from build123d import *

# Parameters (mm, degrees)
SKETCH1_W           = 75
SKETCH1_H           = 75
SKETCH1_R           = 2.625
BOSS_EXTRUDE1_DEPTH = 6.35
FILLET1_R           = 10
SKETCH3_R           = 11.5
SKETCH3_R_2         = 1.75
CUT_EXTRUDE2_DEPTH  = 7.35
SKETCH4_R           = 1.6
CUT_EXTRUDE3_DEPTH  = 7.35


with BuildPart() as part:
    # Sketch1 → Boss-Extrude1 (new body)
    with BuildSketch(Plane(origin=(0, 0, 0), x_dir=(1, 0, 0), z_dir=(0, 1, 0))):
        with Locations((37.5, -37.5)):
            Rectangle(SKETCH1_W, SKETCH1_H)
        with Locations((10, -10)):
            Circle(SKETCH1_R, mode=Mode.SUBTRACT)
        with Locations((45, -10)):
            Circle(SKETCH1_R, mode=Mode.SUBTRACT)
        with Locations((65, -10)):
            Circle(SKETCH1_R, mode=Mode.SUBTRACT)
        with Locations((30, -10)):
            Circle(SKETCH1_R, mode=Mode.SUBTRACT)
    extrude(amount=BOSS_EXTRUDE1_DEPTH)

    # Fillet1
    fillet1_edges = [part.edges().sort_by_distance(p)[0] for p in [
        (75, 3.175, 75),
    ]]
    fillet(fillet1_edges, radius=FILLET1_R)

    # Sketch3 → Cut-Extrude2 (cut, through all)
    with BuildSketch(Plane(origin=(0, 6.35, 0), x_dir=(1, 0, 0), z_dir=(0, 1, 0))):
        with Locations((50, -48)):
            Circle(SKETCH3_R)
        with Locations((34.5, -32.5)):
            Circle(SKETCH3_R_2)
        with Locations((65.5, -32.5)):
            Circle(SKETCH3_R_2)
        with Locations((65.5, -63.5)):
            Circle(SKETCH3_R_2)
        with Locations((34.5, -63.5)):
            Circle(SKETCH3_R_2)
    extrude(amount=-CUT_EXTRUDE2_DEPTH, mode=Mode.SUBTRACT)

    # Sketch4 → Cut-Extrude3 (cut, through all)
    with BuildSketch(Plane(origin=(0, 6.35, 0), x_dir=(1, 0, 0), z_dir=(0, 1, 0))):
        with Locations((22, -15)):
            Circle(SKETCH4_R)
        with Locations((22, -30)):
            Circle(SKETCH4_R)
        with Locations((22, -45)):
            Circle(SKETCH4_R)
        with Locations((22, -60)):
            Circle(SKETCH4_R)
    extrude(amount=-CUT_EXTRUDE3_DEPTH, mode=Mode.SUBTRACT)


solid = part.part
Here's how the part is built. I have some questions about the finished solid (model axes, mm). Round coordinates to 2 decimals unless told otherwise and drop trailing zeros. Order: outer loops, then holes, each group sorted by start corner. A loop starts at its lowest first (then second) coordinate and runs counter-clockwise, first axis right, second up. Notation, with made-up numbers: (16, 83) -> (57, 83) arc R16 cw to (57, 102) -> close; hole circle Ø8 at (-39.75, -8). An arc over 180 degrees is marked (long way). Return JSON: item names as keys, results as strings.
Q1. If we section it at C-C on z = 48: List the corners of the cut face in (x, y) for me, plus the area to 3 significant figures.
Filled sheet:
{"outline": "(0, 0) -> (38.5, 0) -> (38.5, 6.35) -> (0, 6.35) -> close; (61.5, 0) -> (75, 0) -> (75, 6.35) -> (61.5, 6.35) -> close", "area": "330 mm^2"}
Q2. For pin 1 Ø4.5 at (x, z) = (45, 10) entering from -Y (1 decimal), with a flat end and sliding along its axis, tell me the tip position at first contact or that it passes through.
Filled sheet:
{"pin 1": "passes through"}
Q3. If we section it at B-B on z = 10: List the corners of the cut face in (x, y) for me (3 decimals).
Filled sheet:
{"outline": "(0, 0) -> (7.375, 0) -> (7.375, 6.35) -> (0, 6.35) -> close; (12.625, 0) -> (27.375, 0) -> (27.375, 6.35) -> (12.625, 6.35) -> close; (32.625, 0) -> (42.375, 0) -> (42.375, 6.35) -> (32.625, 6.35) -> close; (47.625, 0) -> (62.375, 0) -> (62.375, 6.35) -> (47.625, 6.35) -> close; (67.625, 0) -> (75, 0) -> (75, 6.35) -> (67.625, 6.35) -> close"}
Q4. If we section it at D-D on x = 22: List the corners of the cut face in (y, z) for me, plus the area to 3 significant figures.
Filled sheet:
{"outline": "(0, 0) -> (6.35, 0) -> (6.35, 13.4) -> (0, 13.4) -> close; (0, 16.6) -> (6.35, 16.6) -> (6.35, 28.4) -> (0, 28.4) -> close; (0, 31.6) -> (6.35, 31.6) -> (6.35, 43.4) -> (0, 43.4) -> close; (0, 46.6) -> (6.35, 46.6) -> (6.35, 58.4) -> (0, 58.4) -> close; (0, 61.6) -> (6.35, 61.6) -> (6.35, 75) -> (0, 75) -> close", "area": "395 mm^2"}
Q5. I need wall thicknesses on line 1 along X through (y, z) = (4, 63.5); line 2 along Z through (x, y) = (22, 5.25); line 3 along X through (y, z) = (5.25, 10) (3 decimals). Which ranges of each line are inside material? Lowest first, please. Write a range as from..to.
Filled sheet:
{"line 1": "x = 0..32.75, 36.25..63.75, 67.25..75", "line 2": "z = 0..13.4, 16.6..28.4, 31.6..43.4, 46.6..58.4, 61.6..75", "line 3": "x = 0..7.375, 12.625..27.375, 32.625..42.375, 47.625..62.375, 67.625..75"}
Q6. If we section it at A-A on x = 34.5: List the corners of the cut face in (y, z) for me, plus the area to 3 significant figures.
Filled sheet:
{"outline": "(0, 0) -> (6.35, 0) -> (6.35, 30.75) -> (0, 30.75) -> close; (0, 34.25) -> (6.35, 34.25) -> (6.35, 61.75) -> (0, 61.75) -> close; (0, 65.25) -> (6.35, 65.25) -> (6.35, 75) -> (0, 75) -> close", "area": "432 mm^2"}
Q7. If we mould it in two halves opening along Z, with no side actions, what happens to faces 1 (the flat face through (37, 6.35, 37)), 2 (the cylindrical face through (34.12, 3.22, 65.21)), 3 (the cylindrical face through (71.99, 3.22, 72.15)), 4 (the flat face through (37, 3, 0))? For each: released by +Z, released by -Z, zero draft, split by the parting line, or undercut.
Filled sheet:
{"face 1": "zero draft", "face 2": "undercut", "face 3": "released by +Z", "face 4": "released by -Z"}
